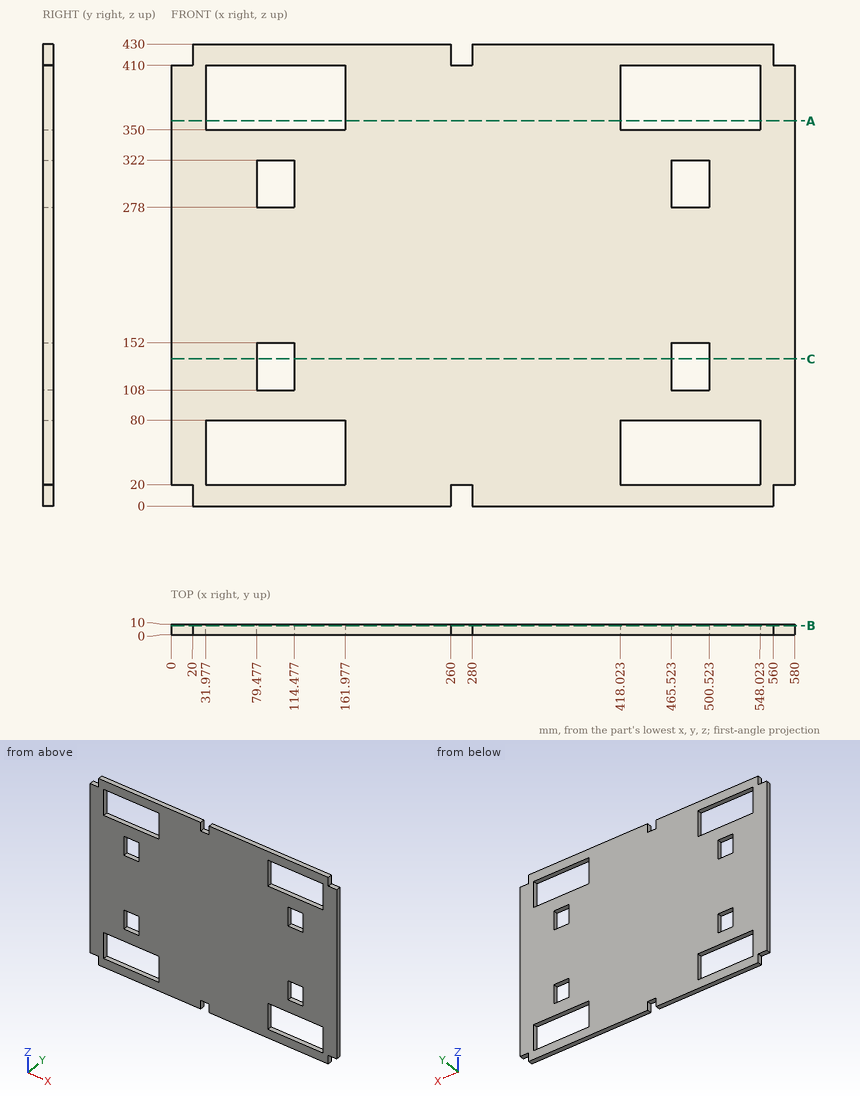
Print and shaded views of the part. All mm, measured from the part's lowest x, y and z. Coordinates: 2 decimals unless noted, no trailing zeros. Write each loop counter-clockwise with the first axis right and the second up, starting at its lowest first coordinate (ties: lowest second). Pieces come first, ordered by that corner, then holes.
(1) Drill centre lines: probe 1 along X at (y, z) = (2.75, 123.5); probe 2 along Z at (x, y) = (491.5, 3.75); probe 3 along Z at (x, y) = (547, 6.25). Where is each one in solid material? Low to high.
(2) Flat gauge pins, fed straight in: pin 1 (3 mm diameter, centred on y = 6.5, z = 93.5, fed in from -X); pin 2 (3 mm diameter, centred on y = 6.5, z = 6, fed in from +X); pin 3 (3 mm diameter, centred on x = 573.5, y = 3.5, fed in from -Z); pin 4 (5 mm diameter, centred on y = 6, z = 425, fed in from -X). Where does each tip first touch, or does it go through?
(3) Cut at A-A, the plane z = 358.5. List the corners of the cut face in (x, y).
(4) Cut at B-B, the plane y = 8.5. Count the separate pieces of the cut face and the enclosed holes in it, and give its area (3 significant figures).
(5) Cut at C-C, the plane z = 137. List the corners of the cut face in (x, y), and give its area (3 significant figures).
Geometry says:
1. probe 1: x = 0 to 79.48, 114.48 to 465.52, 500.52 to 580
1. probe 2: z = 0 to 20, 80 to 108, 152 to 278, 322 to 350, 410 to 430
1. probe 3: z = 0 to 20, 80 to 350, 410 to 430
2. pin 1: stops at x = 0
2. pin 2: stops at x = 560
2. pin 3: stops at z = 20
2. pin 4: stops at x = 20
3. outline: (0, 0) - (31.98, 0) - (31.98, 10) - (0, 10) - close; (161.98, 0) - (418.02, 0) - (418.02, 10) - (161.98, 10) - close; (548.02, 0) - (580, 0) - (580, 10) - (548.02, 10) - close
4. separate pieces: 1
4. enclosed holes: 8
4. area: 210,000 mm2
5. outline: (0, 0) - (79.48, 0) - (79.48, 10) - (0, 10) - close; (114.48, 0) - (465.52, 0) - (465.52, 10) - (114.48, 10) - close; (500.52, 0) - (580, 0) - (580, 10) - (500.52, 10) - close
5. area: 5,100 mm2
